Source: CAD feature listing. Evaluate the final solid. Frame: model axes, mm. Give positions to 0.01 mm unless a question says otherwise; leave off trailing zeros. One line per question, with ' | ' between items. Start each with the question number.
from build123d import *

# Parameters (mm, degrees)
ESQUISSE1_W             = 44.6
ESQUISSE1_H             = 29.3
ESQUISSE1_R             = 1.1
BOSS_EXTRU_2_DEPTH      = 1.2
ENL_V_MAT_EXTRU_1_DEPTH = 0.01


with BuildPart() as part:
    # Esquisse1 → Boss.-Extru.2 (new body)
    with BuildSketch(Plane(origin=(0, 0, 0), x_dir=(1, 0, 0), z_dir=(0, 1, 0))):
        Rectangle(ESQUISSE1_W, ESQUISSE1_H)
        with Locations(Location((16.7, -12.25, 0), (0, 0, 270))):
            Circle(ESQUISSE1_R, mode=Mode.SUBTRACT)
    extrude(amount=BOSS_EXTRU_2_DEPTH)

    # Esquisse7 → Enlèv. mat.-Extru.1 (cut)
    with BuildSketch(Plane(origin=(0, 1.2, 0), x_dir=(1, 0, 0), z_dir=(0, 1, 0))):
        with BuildLine():
            Line((1, 13.65), (7, 13.65))
            ThreePointArc((7, 13.65), (9.4, 9.85), (7, 6.05))
            Line((7, 6.05), (1, 6.05))
            ThreePointArc((1, 6.05), (-1.4, 9.85), (1, 13.65))
        make_face()
        with BuildLine():
            Line((1, -5.3), (7, -5.3))
            ThreePointArc((7, -5.3), (9.4, -9.1), (7, -12.9))
            Line((7, -12.9), (1, -12.9))
            ThreePointArc((1, -12.9), (-1.4, -9.1), (1, -5.3))
        make_face()
        with BuildLine():
            Line((-13.3, 3.375), (-13.3, -2.625))
            ThreePointArc((-13.3, -2.625), (-9.5, -5.025), (-5.7, -2.625))
            Line((-5.7, -2.625), (-5.7, 3.375))
            ThreePointArc((-5.7, 3.375), (-9.5, 5.775), (-13.3, 3.375))
        make_face()
        with BuildLine():
            Line((13.7, 3.375), (13.7, -2.625))
            ThreePointArc((13.7, -2.625), (17.5, -5.025), (21.3, -2.625))
            Line((21.3, -2.625), (21.3, 3.375))
            ThreePointArc((21.3, 3.375), (17.5, 5.775), (13.7, 3.375))
        make_face()
    extrude(amount=-ENL_V_MAT_EXTRU_1_DEPTH, mode=Mode.SUBTRACT)


solid = part.part
Item 1: Mould query, pull axis Z, two halves, no side actions, for faces 1 (the flat face through (0, 1, 14.65)), 2 (the flat face through (-22.3, 1, 0)), 3 (the cylindrical face through (17.79, 0.59, 12.11)). Classes: pulls with the +Z half, pulls with the -Z half, needs draft (parallel to the pull), parting line crosses it, or undercut.
Item 2: Line query: line 1 (X direction, y = 0.9, z = 12.25); line 2 (Y direction, x = 20.5, z = -3.5). Output: solid intervals per line, ascending.
Item 3: Pin query (flat end, axial travel): pin 1 Ø2.5 at (x, z) = (-8.5, 1.5) entering from +Y. Return the tip coordinate at first contact, or that it passes through.
Results are:
1) face 1: pulls with the +Z half | face 2: needs draft | face 3: undercut
2) line 1: x = -22.3 to 15.6, 17.8 to 22.3 | line 2: y = 0 to 1.19
3) pin 1: stops at y = 1.19
